Design review of the part built by this model. Coordinates are the model's own, in mm. A direction names the side the tool comes from. Round coordinates to 2 decimals unless told otherwise and drop trailing zeros. Loops run counter-clockwise (first coordinate to the right, second up) from the corner with the lowest first, then second, coordinate; pieces in that order, holes last. Notation, with made-up numbers: (5.5, 7.25) - (26.5, 7.25) arc R28 ccw to (26.5, 32.25) - close; hole circle Ø11 at (13, -1). An arc over 180 degrees is marked (long way). Return JSON: item names as keys, results as strings. Group by question number.
(1) Clearance check with flat-ended pins moving along their axes: pin 1 (4 mm diameter, centred on y = 19.5, z = 27.5, fed in from +X); pin 2 (1.5 mm diameter, centred on x = 58, y = 66, fed in from -Z); pin 3 (1 mm diameter, centred on y = 97, z = 13, fed in from -X). State where each tip first meets the part, or that it passes through.
(2) For faces 4 (the flat face through (110, 86, 0)), 5 (the flat face through (70, 75, 0)), list the 3-axis set-ups (+Z, -Z, +X, -X, +Y, -Y) from which the entire face can be reached by the end or side of a thin tool; tool diameter is ignored.
(3) Wall thickness on L1, parallel to Y at x = 86, z = 0; L2, parallel to X at y = 103.5, z = 36; L3, parallel to Z at x = 48, y = 95: over which ranges is each line inside the solid? List them lowest first. Write a range as [from, to].
(4) We need section B-B, the plane y = 75. Write out the cut boundary in (x, z), and give its area (3 significant figures).
(5) The part is to be moulded in two halves that separate along Z. For faces 1 (the cylindrical face through (90.28, 84.915, 1.302)), 2 (the cylindrical face through (69.955, 64.487, 33.384)), 3 (the flat face through (0, 120, 0)), say which applies: pulls with the +Z half, pulls with the -Z half, needs draft (parallel to the pull), parting line crosses it, or undercut.
(6) We need section C-C, the plane y = 15.5. Write out the cut boundary in (x, z), and give its area (3 significant figures).
from build123d import *

# Parameters (mm, degrees)
SKETCH1_R           = 42.5
BOSS_EXTRUDE1_DEPTH = 120
SKETCH2_R           = 35
BOSS_EXTRUDE2_DEPTH = 110
FILLET1_R           = 10
SKETCH3_R           = 10
CUT_EXTRUDE1_DEPTH  = 40
FILLET2_R           = 10


with BuildPart() as part:
    # Sketch1 → Boss-Extrude1 (new body)
    with BuildSketch(Plane(origin=(0, 0, 0), x_dir=(1, 0, 0), z_dir=(0, 1, 0))):
        with Locations(Location((0, 0, 0), (0, 0, 90))):
            Circle(SKETCH1_R)
    extrude(amount=BOSS_EXTRUDE1_DEPTH)

    # Sketch2 → Boss-Extrude2 (add)
    with BuildSketch(Plane(origin=(0, 0, 0), x_dir=(0, 0, -1), z_dir=(1, 0, 0))):
        with Locations(Location((0, 75, 0), (0, 0, 180))):
            Circle(SKETCH2_R)
    extrude(amount=BOSS_EXTRUDE2_DEPTH)

    # Fillet1
    fillet1_edges = [part.edges().sort_by_distance(p)[0] for p in [
        (0, 120, 42.5),
    ]]
    fillet(fillet1_edges, radius=FILLET1_R - 0.0001)  # a hair under: the kernel refuses the full size

    # Sketch3 → Cut-Extrude1 (cut)
    with BuildSketch(Plane(origin=(110, 0, 0), x_dir=(0, 0, -1), z_dir=(1, 0, 0))):
        with Locations((0, 75)):
            Circle(SKETCH3_R)
    extrude(amount=-CUT_EXTRUDE1_DEPTH, mode=Mode.SUBTRACT)

    # Fillet2
    fillet2_edges = [part.edges().sort_by_distance(p)[0] for p in [
        (110, 75, -35),
    ]]
    fillet(fillet2_edges, radius=FILLET2_R)


solid = part.part
Solutions:
{
 "1": {"pin 1": "x = 34", "pin 2": "z = -34.01", "pin 3": "x = -40.62"},
 "2": {"face 4": "+Z, -Z, +X, +Y, -Y", "face 5": "+X"},
 "3": {"L1": "[40, 65], [85, 110]", "L2": "[-22.59, 22.59]", "L3": "[-28.72, 28.72]"},
 "4": {"outline": "(24.11, -35) - (100, -35) arc R10 ccw to (110, -25) - (110, -10) - (70, -10) - (70, 10) - (110, 10) - (110, 25) arc R10 ccw to (100, 35) - (24.11, 35) arc R42.5 ccw (long way) to start", "area": "9,940 mm^2"},
 "5": {"face 1": "undercut", "face 2": "parting line crosses it", "face 3": "needs draft"},
 "6": {"outline": "circle Ø85 at (0, 0)", "area": "5,670 mm^2"}
}
